```python
from build123d import *

# Parameters (mm, degrees)
SKETCH1_R           = 58.05
SKETCH1_R_2         = 57.023
BOSS_EXTRUDE1_DEPTH = 13.97
SKETCH2_R           = 59.055
BOSS_EXTRUDE2_DEPTH = 6.35
THREAD1_PITCH       = 3.175
FILLET1_R           = 1.27
FILLET2_R           = 15
SKETCH3_W           = 28
SKETCH3_H           = 8.5
CUT_EXTRUDE1_DEPTH  = 10


with BuildPart() as part:
    # Sketch1 → Boss-Extrude1 (new body)
    with BuildSketch(Plane(origin=(0, 0, 0), x_dir=(1, 0, 0), z_dir=(0, 1, 0))):
        with Locations(Location((0, 0, 0), (0, 0, 270))):
            Circle(SKETCH1_R)
        with Locations(Location((0, 0, 0), (0, 0, 270))):
            Circle(SKETCH1_R_2, mode=Mode.SUBTRACT)
    extrude(amount=BOSS_EXTRUDE1_DEPTH)

    # Sketch2 → Boss-Extrude2 (add)
    with BuildSketch(Plane(origin=(0, 13.97, 0), x_dir=(1, 0, 0), z_dir=(0, 1, 0))):
        with Locations(Location((0, 0, 0), (0, 0, 270))):
            Circle(SKETCH2_R)
    extrude(amount=BOSS_EXTRUDE2_DEPTH)

    # Thread1: arcs per turn and ends read off the stored shape
    # Thread1: the profile of Thread Profile3 profile screwed along a right-hand helix through 2 turns, 12 arcs to a turn; built about Z, then put on its axis
    thread1_z = Axis((0, 0, 0), (0, 0, 1))
    thread1_corners = [(57.0233, 2.5e-08, -0.000173205), (57.0233, 2.5e-08, 2.778298196), (55.304480847, 2.4e-08, 1.785937496), (55.304480847, 2.4e-08, 0.992187496)]
    with BuildLine(mode=Mode.PRIVATE) as thread1_profile:
        Line(thread1_corners[0], thread1_corners[1])
        Line(thread1_corners[1], thread1_corners[2])
        Line(thread1_corners[2], thread1_corners[3])
        Line(thread1_corners[3], thread1_corners[0])
    thread1_cap = Face(thread1_profile.wire())
    thread1_turn_angles = [0, 15, 30, 45, 60, 75, 90, 105, 120, 135, 150, 165, 180, 195, 210, 225, 240, 255, 270, 285, 300, 315, 330, 345, 360]
    thread1_turn_weights = [1, 0.9659258262890683, 1, 0.9659258262890683, 1, 0.9659258262890683, 1, 0.9659258262890683, 1, 0.9659258262890683, 1, 0.9659258262890683, 1, 0.9659258262890683, 1, 0.9659258262890683, 1, 0.9659258262890683, 1, 0.9659258262890683, 1, 0.9659258262890683, 1, 0.9659258262890683, 1]
    thread1_turn_rails = [Edge.make_bspline([Vector(p[0], p[1], 0).rotate(thread1_z, thread1_turn_angles[k]) / thread1_turn_weights[k] + Vector(0, 0, p[2] + THREAD1_PITCH * thread1_turn_angles[k] / 360) for k in range(25)], [0, 0, 0, 1, 1, 2, 2, 3, 3, 4, 4, 5, 5, 6, 6, 7, 7, 8, 8, 9, 9, 10, 10, 11, 11, 12, 12, 12], 2, thread1_turn_weights) for p in thread1_corners]
    thread1_turn_sides = [Face.make_surface_from_curves(thread1_turn_rails[p[0]], thread1_turn_rails[p[1]]) for p in [(0, 1), (1, 2), (2, 3), (3, 0)]]
    thread1 = Plane(origin=(0, 13.97, 0), x_dir=(-0.999847695, 0, -0.017452406), z_dir=(0, -1, 0)) * Solid(Shell([*[p.moved(Location((0, 0, THREAD1_PITCH * i))) for i in range(2) for p in thread1_turn_sides], thread1_cap, thread1_cap.rotate(thread1_z, 720).moved(Location((0, 0, THREAD1_PITCH * 720 / 360)))]))
    add(thread1)

    # Fillet1
    fillet1_edges = [part.edges().sort_by_distance(p)[0] for p in [
        (0, 20.32, -59.055),
    ]]
    fillet(fillet1_edges, radius=FILLET1_R)

    # Fillet2
    # the kernel refuses this fillet: 15 mm, written as the material it adds along each edge
    with BuildSketch(Plane(origin=(0, 13.97, 0), x_dir=(0, 0, 1), z_dir=(-1, 0, 0))) as fillet2_piece_1:
        with BuildLine():
            CenterArc((73.05, -5.398145515), FILLET2_R, 158.907396465, 21.092603535)
            Line((58.05, -5.398145515), (57.75, -5.398145515))
            Line((57.75, -5.398145515), (57.75, 0))
            Line((57.75, 0), (58.05, 0.3))
            ThreePointArc((58.05, 0.3), (58.5525, 0.3), (58.7751, 0.10796291))
            Line((58.7751, 0.10796291), (59.055, 0))
        make_face()
    revolve(axis=Axis((0, 13.97, 0), (0, 1, 0)))

    # Sketch3 → Cut-Extrude1 (cut)
    with BuildSketch(Plane(origin=(0, 20.32, 0), x_dir=(1, 0, 0), z_dir=(0, 1, 0))):
        with BuildLine():
            Line((-28, -8.5), (-28, 0))
            Line((-28, 0), (-36.5, 0))
            ThreePointArc((-36.5, 0), (-34.01040764, -6.01040764), (-28, -8.5))
        make_face()
        with BuildLine():
            Line((-36.5, 0), (-28, 0))
            Line((-28, 0), (-28, 8.5))
            ThreePointArc((-28, 8.5), (-34.01040764, 6.01040764), (-36.5, 0))
        make_face()
        with Locations((-14, 4.25)):
            Rectangle(SKETCH3_W, SKETCH3_H)
        Polygon((0, 8.5), (0, 0), (-28, 0), (-28, -8.5), (28, -8.5), (28, 8.5), align=None)
        with BuildLine():
            ThreePointArc((28, 8.5), (36.5, 0), (28, -8.5))
            Line((28, -8.5), (28, 8.5))
        make_face()
    extrude(amount=-CUT_EXTRUDE1_DEPTH, mode=Mode.SUBTRACT)


solid = part.part
```
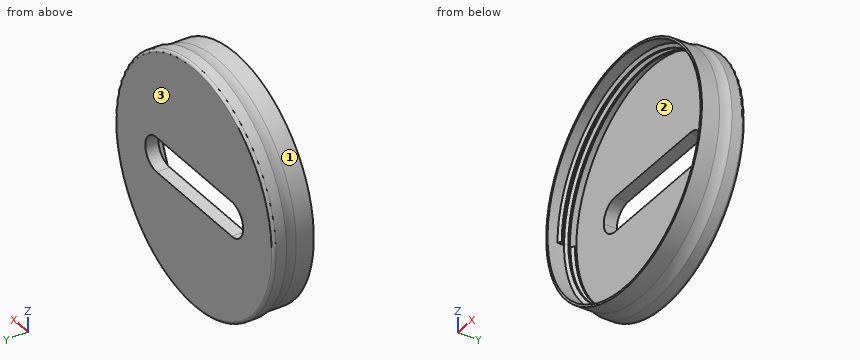
Work out the finished part from the listing and answer in its coordinate system (mm). Face numbers are marked on the shaded views. Give positions to 0.01 mm unless a question says otherwise; leave off trailing zeros. Use one line per item in the form item = value.
1. Determine the mould class of the marked faces 1, 2 and 3 for opening direction Z: released by +Z, released by -Z, zero draft, split by the parting line, or undercut.
Filled in:
face_1 = split by the parting line
face_2 = undercut
face_3 = zero draft
2. Consider L1, parallel to X at y = 2.5, z = 0; L2, parallel to Y at x = -9, z = 34; L3, parallel to X at y = 12.8, z = 0. Determine where each line is inside the solid, lowest interval first.
Filled in:
L1 = -58.05 to -57.02, 57.02 to 58.05
L2 = 13.97 to 20.32
L3 = -58.66 to -57.02, 57.02 to 58.66
3. Each of these flat-tipped pins is pushed along its axis until it touches: pin 1 Ø10 at (x, z) = (7, 14.5) entering from -Y; pin 2 Ø6 at (x, y) = (-45, 10) entering from -Z; pin 3 Ø8 at (x, y) = (-24.5, 4.5) entering from -Z. Where does it stop, or does it pass through?
Filled in:
pin_1 = 13.97
pin_2 = -40.21
pin_3 = -54.31
